Here's how the part is built. I have some questions about the finished solid (model axes, mm). Face numbers are marked on the shaded views. A direction names the side the tool comes from. Give positions to 0.01 mm unless a question says otherwise; leave off trailing zeros. Write each loop counter-clockwise with the first axis right and the second up, starting at its lowest first coordinate (ties: lowest second). Pieces come first, ordered by that corner, then holes. Notation, with made-up numbers: (78, 72.5) -> (113, 72.5) arc R27 cw to (113, 96.5) -> close; hole circle Ø10 at (-24.75, 53.25). An arc over 180 degrees is marked (long way). Use CSV: the item, a comma, the result in double quotes. Start each with the question number.
(1) For pin 1 Ø1 at (x, y) = (26, 2.5) entering from +Z; pin 2 Ø25 at (x, y) = (-2.5, -1.5) entering from +Z; pin 3 Ø5 at (x, z) = (-28.5, -10) entering from -Y, each with a flat end and sliding along its axis, tell me the tip position at first contact or that it passes through.
(2) Suppose I cut it at B-B on y = 9.5. List the corners of the cut face in (x, z) for me.
(3) Which directions (+Z, -Z, +X, -X, +Y, -Y) give clear straight access to the entire face, cutting with the end or side of a thin tool? Please do the marked faces 1 and 2.
(4) I need wall thicknesses on L1, parallel to X at y = 9, z = -10; L2, parallel to Z at x = 28.5, y = 16.5; L3, parallel to X at y = -22, z = -8. Which ranges of each line are inside material? Lowest first, please. Write a range as [from, to].
(5) Suppose I cut it at C-C on x = -28.5. List the corners of the cut face in (y, z) for me, plus the area to 3 significant figures.
(6) Suppose I cut it at A-A on z = -12.5. List the corners of the cut face in (x, y) for me.
(7) Suppose I cut it at D-D on x = 21. List the corners of the cut face in (y, z) for me.
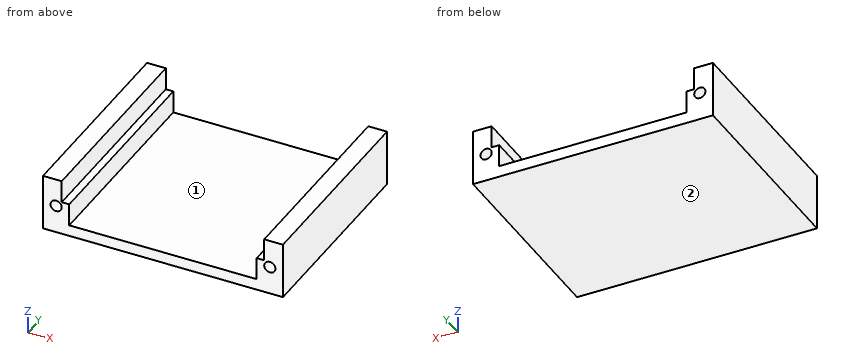
from build123d import *

# Parameters (mm, degrees)
SKETCH004_W             = 64
SKETCH004_H             = 54
PAD002_DEPTH            = 3
SKETCH005_W             = 7
SKETCH005_H             = 54
PAD003_DEPTH            = 12
SKETCH008_R             = 1.5
POCKET003_DEPTH         = 60
SKETCH009_R             = 1.5
POCKET004_DEPTH         = 60
SKETCH016_W             = 54
SKETCH016_H             = 6
POCKET008_DEPTH         = 2
SKETCH017_W             = 54
SKETCH017_H             = 6
POCKET009_DEPTH         = 2
BODY001_PLACEMENT_ANGLE = 180


with BuildPart() as part:
    # Sketch004 → Pad002 (new body)
    with BuildSketch(Plane.XY):
        Rectangle(SKETCH004_W, SKETCH004_H)
    extrude(amount=PAD002_DEPTH)

    # Sketch005 (on Face5 of Pad002) → Pad003 (join)
    with BuildSketch(Plane(origin=(0, 0, 0), x_dir=(1, 0, 0), z_dir=(0, 0, -1))):
        with Locations((28.5, 0)):
            Rectangle(SKETCH005_W, SKETCH005_H)
        with Locations((-28.5, 0)):
            Rectangle(SKETCH005_W, SKETCH005_H)
    extrude(amount=PAD003_DEPTH)

    # Sketch008 (on Face15 of Pad003) → Pocket003 (cut)
    with BuildSketch(Plane.XZ.offset(27)):
        with Locations((28.5, -4.5)):
            Circle(SKETCH008_R)
    extrude(amount=-POCKET003_DEPTH, mode=Mode.SUBTRACT)

    # Sketch009 (on Face16 of Pocket003) → Pocket004 (cut)
    with BuildSketch(Plane.XZ.offset(27)):
        with Locations((-28.5, -4.5)):
            Circle(SKETCH009_R)
    extrude(amount=-POCKET004_DEPTH, mode=Mode.SUBTRACT)

    # Sketch016 (on Face11 of Pocket004) → Pocket008 (cut)
    with BuildSketch(Plane.YZ.offset(-25)):
        with Locations((0, -9)):
            Rectangle(SKETCH016_W, SKETCH016_H)
    extrude(amount=-POCKET008_DEPTH, mode=Mode.SUBTRACT)

    # Sketch017 (on Face16 of Pocket008) → Pocket009 (cut)
    with BuildSketch(Plane(origin=(25, 0, 0), x_dir=(0, -1, 0), z_dir=(-1, 0, 0))):
        with Locations((0, -9)):
            Rectangle(SKETCH017_W, SKETCH017_H)
    extrude(amount=-POCKET009_DEPTH, mode=Mode.SUBTRACT)


with BuildPart() as part_1:
    # Body001 placement: moved
    add(part.part.moved(Location((0, 0, -14.5))).rotate(Axis((0, 0, -14.5), (1, 0, 0)), BODY001_PLACEMENT_ANGLE))


solid = part_1.part
Geometry says:
1,pin 1,"z = -8.5"
1,pin 2,"z = -14.5"
1,pin 3,"y = -27"
2,outline,"(-32, -17.5) -> (32, -17.5) -> (32, -2.5) -> (27, -2.5) -> (27, -8.5) -> (25, -8.5) -> (25, -14.5) -> (-25, -14.5) -> (-25, -8.5) -> (-27, -8.5) -> (-27, -2.5) -> (-32, -2.5) -> close; hole circle Ø3 at (-28.5, -10); hole circle Ø3 at (28.5, -10)"
3,face 1,"+Z, +Y, -Y"
3,face 2,"-Z, +X, -X, +Y, -Y"
4,L1,"[-32, -30], [-27, -25], [25, 27], [30, 32]"
4,L2,"[-17.5, -11.5], [-8.5, -2.5]"
4,L3,"[-32, -27], [27, 32]"
5,outline,"(-27, -17.5) -> (27, -17.5) -> (27, -11.5) -> (-27, -11.5) -> close; (-27, -8.5) -> (27, -8.5) -> (27, -2.5) -> (-27, -2.5) -> close"
5,area,"648 mm²"
6,outline,"(-32, -27) -> (-25, -27) -> (-25, 27) -> (-32, 27) -> close; (25, -27) -> (32, -27) -> (32, 27) -> (25, 27) -> close"
7,outline,"(-27, -17.5) -> (27, -17.5) -> (27, -14.5) -> (-27, -14.5) -> close"
